Input: part model. Units: mm. Frame: model coordinates. A direction names the side the tool comes from. Coordinates: 2 decimals unless noted, no trailing zeros. Order: outer loops, then holes, each group sorted by start corner. A loop starts at its lowest first (then second) coordinate and runs counter-clockwise, first axis right, second up.
Autodesk Inventor part; units mm, degrees
ref_plane "YZ Plane" through (0, 0, 0) normal (1, 0, 0) x (0, 1, 0)
ref_plane "XZ Plane" through (0, 0, 0) normal (0, 1, 0) x (-1, 0, 0)
ref_plane "XY Plane" through (0, 0, 0) normal (0, 0, 1) x (1, 0, 0)
sketch "Sketch1" plane through (0, 0, 0) normal (1, 0, 0) x (0, 1, 0)
  arc A0 (0, 22) -> (0, 0) centre (0, 11) ccw
  line L0 (-11, 11) -> (24, 11) construction
  arc A1 (35.1478, 22) -> (35.1478, 0) centre (35.1478, 11) ccw
  arc A2 (0, 27) -> (0, -5) centre (0, 11) ccw
  line L1 (0, -5) -> (58, -5)
  arc A3 (35.1478, 5022) -> (35.1478, -5000) centre (35.1478, 11) ccw
  arc A4 (35.1478, 27) -> (19.1478, 11) centre (35.1478, 11) ccw
  line L2 (0, 0) -> (14.1478, 0)
  line L3 (35.1478, 0) -> (58, 0)
  line L4 (35.1478, 27) -> (40.1478, 27)
  line L5 (42.1478, 25) -> (42.1478, 24)
  line L6 (40.1478, 22) -> (35.1478, 22)
  line L7 (0, 27) -> (5, 27)
  line L8 (7, 25) -> (7, 24)
  line L9 (5, 22) -> (0, 22)
  line L10 (60, -2) -> (60, -3)
  arc A5 (40.1478, 22) -> (42.1478, 24) centre (40.1478, 24) ccw
  arc A6 (42.1478, 25) -> (40.1478, 27) centre (40.1478, 25) ccw
  arc A7 (60, -2) -> (58, 0) centre (58, -2) ccw
  arc A8 (58, -5) -> (60, -3) centre (58, -3) ccw
  arc A9 (5, 22) -> (7, 24) centre (5, 24) ccw
  arc A10 (7, 25) -> (5, 27) centre (5, 25) ccw
  line L11 (19.1478, 11) -> (19.1478, 5)
  arc A11 (14.1478, 0) -> (19.1478, 5) centre (14.1478, 5) ccw
  point P0 (60, 0)
  point P1 (42.1478, 27)
  point P2 (42.1478, 22)
  point P3 (7, 27)
  dimension "d0" = 60
  dimension "d1" = 22
  dimension "d2" = 35
  dimension "d3" = 22
  dimension "d5" = 5
  dimension "d6" = 5000
  dimension "d7" = 5
  dimension "d8" = 7
  dimension "d9" = 5
  dimension "d10" = 7
  dimension "d11" = 2
  dimension "d12" = 5
extrude "Extrusion1" add sketch "Sketch1" along normal blind 8
ref_plane "Work Plane1" through (2, 58, 0) normal (0, 0, 1) x (1, 0, 0)
sketch "Sketch2" plane through (2, 58, 0) normal (0, 0, 1) x (1, 0, 0)
  line L0 (-2, 0) -> (6, 0) construction
  line L1 (-2, -22.8522) -> (6, -22.8522) construction
  line L2 (0, 0) -> (4, 0) construction
  line L3 (2, 0) -> (2, -9.8019) construction
  line L4 (-2, 0) -> (-2, -22.8522)
  line L5 (6, 0) -> (6, -22.8522)
  point P0 (-2, -58)
  point P1 (2, -4.901)
hole "Hole1" at (4, 53.099, 0) direction (0, 0, -1) diameter 5 end through all countersink diameter 7 countersink angle 90
properties part number "double_rounded_slim"
Item 1: Ray query, probe 1 along Z at (x, y) = (2, -0.5); probe 2 along Z at (x, y) = (1, 10); probe 3 along Y at (x, z) = (5.25, 11.5). Return the intervals inside material, ascending.
Response values:
probe 1: z = -4.99 to 0.01, 21.99 to 26.99
probe 2: z = -5 to 0
probe 3: y = -15.99 to -10.99, 19.16 to 24.16
Item 2: Access query for faces 5 (the face through (3.944, 41.577, 22.601)), 6 (the face through (4, 2, 27)), 7 (the face through (4, 19.148, 8)), 8 (the face through (4, 3, 22)). Directions: +Z, -Z, +X, -X, +Y, -Y. A direction counts if a zero-diameter tool reaches every point of the face in a straight line with its end or side. Return the directions, or none.
Response values:
face 5: +X, -X, +Y
face 6: +Z, +X, -X, +Y, -Y
face 7: +Z, +X, -X
face 8: +X, -X
Item 3: Cut plane C-C on y = -3. Return loops of the section in (x, z), then the cut area to 3 significant figures.
Response values:
outline: (0, -4.72) - (8, -4.72) - (8, 0.42) - (0, 0.42) - close; (0, 21.58) - (8, 21.58) - (8, 26.72) - (0, 26.72) - close
area: 82.1 mm2
Item 4: Pin query (flat end, axial travel): pin 1 Ø3 at (y, z) = (-3, 19.5) entering from -X; pin 2 Ø1.8 at (x, z) = (4.5, 8) entering from -Y; pin 3 Ø3 at (x, y) = (3, -1) entering from +Z; pin 4 Ø0.8 at (x, z) = (3.5, 24.5) entering from +Y. Return the tip coordinate at first contact, or that it passes through.
Response values:
pin 1: passes through
pin 2: stops at y = -15.86
pin 3: stops at z = 27
pin 4: stops at y = 42.15
Item 5: Cut plane D-D on y = 22. Return loops of the section in (x, z), then the cut area to 3 significant figures.
Response values:
outline: (0, -5) - (8, -5) - (8, 20.12) - (0, 20.12) - close
area: 201 mm2
Item 6: Cut plane B-B on z = 23. Return loops of the section in (x, y).
Response values:
outline: (0, -10.58) - (8, -10.58) - (8, 6.73) - (0, 6.73) - close; (0, 24.56) - (8, 24.56) - (8, 41.88) - (0, 41.88) - close
Item 7: Cut plane A-A on x = 4. Return loops of the section in (y, z), then the cut area to 3 significant figures.
Response values:
outline: (0, -5) - (50.6, -5) - (50.6, -1) - (49.6, 0) - (35.15, 0) arc R11 cw to (35.15, 22) - (40.15, 22) arc R2 ccw to (42.15, 24) - (42.15, 25) arc R2 ccw to (40.15, 27) - (35.15, 27) arc R16 ccw to (19.15, 11) - (19.15, 5) arc R5 cw to (14.15, 0) - (0, 0) arc R11 cw to (0, 22) - (5, 22) arc R2 ccw to (7, 24) - (7, 25) arc R2 ccw to (5, 27) - (0, 27) arc R16 ccw to start; (55.6, -5) - (58, -5) arc R2 ccw to (60, -3) - (60, -2) arc R2 ccw to (58, 0) - (56.6, 0) - (55.6, -1) - close
area: 743 mm2
Item 8: Draft query along Z for faces 1 (the face through (3.94, 59.4, -0.57)), 2 (the face through (3.94, 24.15, 10.76)), 3 (the face through (4, 38, 22)), 4 (the face through (4, 29, -5)). Return one class per face: pulls with the +Z half, pulls with the -Z half, needs draft (parallel to the pull), parting line crosses it, or undercut.
Response values:
face 1: pulls with the +Z half
face 2: undercut
face 3: undercut
face 4: pulls with the -Z half
